from build123d import *

# Parameters (mm, degrees)
SKETCH1_W           = 330.2
SKETCH1_H           = 901.7
BOSS_EXTRUDE1_DEPTH = 12.7
SKETCH2_W           = 101.6
SKETCH2_H           = 152.4
CUT_EXTRUDE1_DEPTH  = 7.62
SKETCH3_W           = 50.8
SKETCH3_H           = 50.8
CUT_EXTRUDE2_DEPTH  = 961.341720431
CAVITY1_START       = 66.091277654
CAVITY1_OUTLINE_W   = 12.7
CAVITY1_OUTLINE_H   = 6.301813258
CAVITY1_DEPTH       = 192.893313571


# Read off the part's stored shape, not the designer's step: Cavity1
with BuildPart() as part:
    # Sketch1 → Boss-Extrude1 (new body)
    with BuildSketch(Plane.XY):
        with Locations((165.1, 450.85)):
            Rectangle(SKETCH1_W, SKETCH1_H)
    extrude(amount=BOSS_EXTRUDE1_DEPTH)

    # Sketch2 → Cut-Extrude1 (cut)
    with BuildSketch(Plane.XY.offset(12.7)):
        with Locations((165.1, 698.5)):
            Rectangle(SKETCH2_W, SKETCH2_H)
    extrude(amount=-CUT_EXTRUDE1_DEPTH, mode=Mode.SUBTRACT)

    # Sketch3 → Cut-Extrude2 (cut, through all)
    with BuildSketch(Plane.XY.offset(12.7)):
        with Locations((165.1, 76.2)):
            Rectangle(SKETCH3_W, SKETCH3_H)
    extrude(amount=-CUT_EXTRUDE2_DEPTH, mode=Mode.SUBTRACT)

    # Cavity1 outline → Cavity1 (cut)
    with BuildSketch(Plane.YZ.offset(CAVITY1_START)):
        with Locations((203.2, 9.549093371)):
            Rectangle(CAVITY1_OUTLINE_W, CAVITY1_OUTLINE_H)
    extrude(amount=CAVITY1_DEPTH, mode=Mode.SUBTRACT)


solid = part.part
Check sheet for the modelled part. Datum: model origin and axes. Units: mm. Coordinates: 2 decimals unless noted, no trailing zeros. Loops run counter-clockwise (first coordinate to the right, second up) from the corner with the lowest first, then second, coordinate; pieces in that order, holes last. Notation, with made-up numbers: (-39, 55.25) -> (-33, 55.25) arc R22 ccw to (-33, 73.25) -> close; hole circle Ø4 at (67, -5). An arc over 180 degrees is marked (long way). Write item = value, one per line. Start each with the question number.
1. Section check B-B on y = 74.5. Record the cut outline in (x, z).
2. Draft check along X on faces 1 (the flat face through (164, 700, 5.08)), 2 (the flat face through (163, 457, 12.7)). Enter one of: released by +X, released by -X, zero draft, split by the parting line, or undercut.
3. Material ranges on line 1 (Y direction, x = 131, z = 9.75); line 2 (Y direction, x = 179.5, z = 7.5); line 3 (X direction, y = 99, z = 8), recorded low to high.
4. Section check D-D on y = 746.5. Record the cut outline in (x, z).
5. Section check A-A on x = 172. Record the cut outline in (y, z).
6. Section check C-C on z = 9. Record the cut outline in (x, y).
Responses:
q1.outline = (0, 0) -> (139.7, 0) -> (139.7, 12.7) -> (0, 12.7) -> close; (190.5, 0) -> (330.2, 0) -> (330.2, 12.7) -> (190.5, 12.7) -> close
q2.face_1 = undercut
q2.face_2 = zero draft
q3.line_1 = 0 to 196.85, 209.55 to 622.3, 774.7 to 901.7
q3.line_2 = 0 to 50.8, 101.6 to 196.85, 209.55 to 622.3, 774.7 to 901.7
q3.line_3 = 0 to 139.7, 190.5 to 330.2
q4.outline = (0, 0) -> (330.2, 0) -> (330.2, 12.7) -> (215.9, 12.7) -> (215.9, 5.08) -> (114.3, 5.08) -> (114.3, 12.7) -> (0, 12.7) -> close
q5.outline = (0, 0) -> (50.8, 0) -> (50.8, 12.7) -> (0, 12.7) -> close; (101.6, 0) -> (901.7, 0) -> (901.7, 12.7) -> (774.7, 12.7) -> (774.7, 5.08) -> (622.3, 5.08) -> (622.3, 12.7) -> (209.55, 12.7) -> (209.55, 6.4) -> (196.85, 6.4) -> (196.85, 12.7) -> (101.6, 12.7) -> close
q6.outline = (0, 0) -> (330.2, 0) -> (330.2, 901.7) -> (0, 901.7) -> close; hole (66.09, 196.85) -> (258.98, 196.85) -> (258.98, 209.55) -> (66.09, 209.55) -> close; hole (114.3, 622.3) -> (215.9, 622.3) -> (215.9, 774.7) -> (114.3, 774.7) -> close; hole (139.7, 50.8) -> (190.5, 50.8) -> (190.5, 101.6) -> (139.7, 101.6) -> close
